from build123d import *

# Parameters (mm, degrees)
SKETCH2_W            = 12.8
SKETCH2_H            = 5.8
BOSS_EXTRUDE1_DEPTH  = 6.22
M2_CLEARANCE_HOLE1_D = 2.2
BOSS_EXTRUDE2_DEPTH  = 5.8
SKETCH17_W           = 0.9
SKETCH17_H           = 0.6
BOSS_EXTRUDE3_DEPTH  = 3.7
BOSS_EXTRUDE5_DEPTH  = 3.1


with BuildPart() as part:
    # Sketch2 → Boss-Extrude1 (new body)
    with BuildSketch(Plane.XY):
        with Locations((-6.4, 2.9)):
            Rectangle(SKETCH2_W, SKETCH2_H)
    extrude(amount=BOSS_EXTRUDE1_DEPTH)

    # M2 Clearance Hole1 (through all)
    with Locations(Plane(origin=(0, 0, 0), x_dir=(-1, 0, 0), z_dir=(0, -1, 0))):
        with Locations((9.65, -5.1), (3.15, -5.1)):
            Hole(M2_CLEARANCE_HOLE1_D / 2)

    # Sketch16 → Boss-Extrude2 (add, through all)
    with BuildSketch(Plane.XZ):
        with BuildLine():
            Line((-10.670208312, 6.22), (-8.629791688, 6.22))
            ThreePointArc((-8.629791688, 6.22), (-9.65, 6.615), (-10.670208312, 6.22))
        make_face()
        with BuildLine():
            Line((-4.170208312, 6.22), (-2.129791688, 6.22))
            ThreePointArc((-2.129791688, 6.22), (-3.15, 6.615), (-4.170208312, 6.22))
        make_face()
    extrude(amount=-BOSS_EXTRUDE2_DEPTH)

    # Sketch17 → Boss-Extrude3 (add)
    with BuildSketch(Plane.XY.offset(6.22)):
        with Locations((-6.4, 2.9)):
            Rectangle(SKETCH17_W, SKETCH17_H)
        with Locations((-11.55, 2.9)):
            Rectangle(SKETCH17_W, SKETCH17_H)
        with Locations((-1.25, 2.8)):
            Rectangle(SKETCH17_W, SKETCH17_H)
    extrude(amount=BOSS_EXTRUDE3_DEPTH)

    # Sketch19 → Boss-Extrude5 (add)
    with BuildSketch(Plane(origin=(0, 1.35, 0), x_dir=(1, 0, 0), z_dir=(0, 1, 0))):
        Polygon((-4.3, 1), (-1.452673729, 0), (-1, 0), (-0.547326271, 0), (-0.950295326, 0.141525423), (-14.047326271, 4.741290149), (-14.047326271, 4.423326076), align=None)
    extrude(amount=BOSS_EXTRUDE5_DEPTH)


solid = part.part
Geometry: final body of the model. Coordinates: model frame, mm. A direction names the side the tool comes from. Give positions to 0.01 mm unless a question says otherwise; leave off trailing zeros. Write each loop counter-clockwise with the first axis right and the second up, starting at its lowest first coordinate (ties: lowest second). Pieces come first, ordered by that corner, then holes. Notation, with made-up numbers: (-33, -1) - (3, -1) arc R28 cw to (3, 33) - close; hole circle Ø2 at (36.25, 32). An arc over 180 degrees is marked (long way). Return JSON: item names as keys, results as strings. Group by question number.
1) Section C-C on x = -3.75. Return the cut outline in (y, z), plus the area to 3 significant figures.
2) First-contact query: P1, Ø1.3, axis at x = -3.15, z = 5.1, coming from the +Y side; P2, Ø1, axis at x = -1, z = 8, coming from the -Y side; P3, Ø3, axis at y = 1.5, z = 3.5, coming from the -X side; P4, Ø0.5, axis at y = 3, z = 8, coming from the +X side. Flat tips, straight axial feed; report the tip coordinate or a pass-through.
3) Set-up query: faces 1 (the cylindrical face through (-3.134, 2.859, 6.615)), 2 (the flat face through (-1, 3.1, 8)), 3 (the flat face through (-12.8, 3, 3)), 4 (the flat face through (-11.6, 2.6, 8)). Return all of +Z, -Z, +X, -X, +Y, -Y with unobstructed straight access to the full face (end or side cutting, diameter ignored); none if empty.
4) Section A-A on y = 5.25. Return the cut outline in (x, z) (3 decimals), plus the area to 3 significant figures.
5) Section B-B on z = 5.1. Return the cut outline in (x, y).
6) Section D-D on z = -2.5. Return the cut outline in (x, y), plus the area to 3 significant figures.
7) Line query: line 1 (X direction, y = 3.2, z = 5.1); line 2 (Z direction, x = -3.15, y = 2.6) (3 decimals); line 3 (X direction, y = 2.45, z = 0.75). Output: solid intervals per line, ascending.
Filled in:
{
 "1": {"outline": "(0, 0) - (5.8, 0) - (5.8, 4.18) - (0, 4.18) - close; (0, 6.02) - (5.8, 6.02) - (5.8, 6.49) - (0, 6.49) - close; (1.35, -1.12) - (4.45, -1.12) - (4.45, -0.81) - (1.35, -0.81) - close", "area": "27.9 mm^2"},
 "2": {"P1": "passes through", "P2": "stops at y = 2.5", "P3": "stops at x = -12.8", "P4": "stops at x = -0.8"},
 "3": {"face 1": "+Z, +Y, -Y", "face 2": "+Z, +X, +Y", "face 3": "+Z, -X, +Y, -Y", "face 4": "+Z, -X, -Y"},
 "4": {"outline": "(-12.8, 0) - (0, 0) - (0, 6.22) - (-2.13, 6.22) arc R1.515 ccw to (-4.17, 6.22) - (-8.63, 6.22) arc R1.515 ccw to (-10.67, 6.22) - (-12.8, 6.22) - close; hole circle Ø2.2 at (-9.65, 5.1); hole circle Ø2.2 at (-3.15, 5.1)", "area": "73.1 mm^2"},
 "5": {"outline": "(-12.8, 0) - (-10.75, 0) - (-10.75, 5.8) - (-12.8, 5.8) - close; (-8.55, 0) - (-4.25, 0) - (-4.25, 5.8) - (-8.55, 5.8) - close; (-2.05, 0) - (0, 0) - (0, 5.8) - (-2.05, 5.8) - close"},
 "6": {"outline": "(-8.57, 1.35) - (-7.67, 1.35) - (-7.67, 4.45) - (-8.57, 4.45) - close", "area": "2.81 mm^2"},
 "7": {"line 1": "x = -12.8 to -10.75, -8.55 to -4.25, -2.05 to 0", "line 2": "z = -0.914 to -0.596, 0 to 4, 6.2 to 6.615", "line 3": "x = -12.8 to 0"}
}
